```python
from build123d import *

# Parameters (mm, degrees)
SKETCH_1_R          = 48
SKETCH_1_R_2        = 40
EXTRUDE_1_DEPTH     = 8
SKETCH_2_R          = 45.05
SKETCH_2_R_2        = 42.95
CUT_EXTRUDE_1_DEPTH = 0.5
CUT_EXTRUDE_START   = -7.5
SKETCH_2_2_R        = 45.05
SKETCH_2_2_R_2      = 42.95
CUT_EXTRUDE_2_DEPTH = 0.5
CHAMFER_1_SIZE      = 0.8


with BuildPart() as part:
    # 草图1 → 凸台-拉伸1 (new body)
    with BuildSketch(Plane(origin=(0, 0, 0), x_dir=(1, 0, 0), z_dir=(0, 1, 0))):
        with Locations(Location((0, 0, 0), (0, 0, 270))):
            Circle(SKETCH_1_R)
        with Locations(Location((0, 0, 0), (0, 0, 270))):
            Circle(SKETCH_1_R_2, mode=Mode.SUBTRACT)
    extrude(amount=EXTRUDE_1_DEPTH)

    # 草图2 → 切除-拉伸1 (cut)
    with BuildSketch(Plane(origin=(0, 8, 0), x_dir=(1, 0, 0), z_dir=(0, 1, 0))):
        with Locations(Location((0, 0, 0), (0, 0, 270))):
            Circle(SKETCH_2_R)
        with Locations(Location((0, 0, 0), (0, 0, 270))):
            Circle(SKETCH_2_R_2, mode=Mode.SUBTRACT)
    extrude(amount=-CUT_EXTRUDE_1_DEPTH, mode=Mode.SUBTRACT)

    # 草图2<2> → 切除-拉伸2 (cut)
    with BuildSketch(Plane(origin=(0, 8, 0), x_dir=(1, 0, 0), z_dir=(0, 1, 0)).offset(CUT_EXTRUDE_START)):
        with Locations(Location((0, 0, 0), (0, 0, 270))):
            Circle(SKETCH_2_2_R)
        with Locations(Location((0, 0, 0), (0, 0, 270))):
            Circle(SKETCH_2_2_R_2, mode=Mode.SUBTRACT)
    extrude(amount=-CUT_EXTRUDE_2_DEPTH, mode=Mode.SUBTRACT)

    # 倒角1
    chamfer_1_edges = [part.edges().sort_by_distance(p)[0] for p in [
        (0, 0, -48),
        (0, 8, -48),
        (0, 0, -40),
        (0, 8, -40),
    ]]
    chamfer(chamfer_1_edges, length=CHAMFER_1_SIZE)


solid = part.part
```
Input: part model. Units: mm. Frame: model coordinates. A direction names the side the tool comes from. Round coordinates to 2 decimals unless told otherwise and drop trailing zeros. Order: outer loops, then holes, each group sorted by start corner. A loop starts at its lowest first (then second) coordinate and runs counter-clockwise, first axis right, second up. Notation, with made-up numbers: (58.5, -24) - (116.5, -24) arc R12 ccw to (116.5, -7) - close; hole circle Ø9 at (-17.75, -19.5). An arc over 180 degrees is marked (long way). One line per question, with ' | ' between items. Start each with the question number.
1) Ray query, probe 1 along X at (y, z) = (5, 0); probe 2 along X at (y, z) = (7.8, 0); probe 3 along X at (y, z) = (0.1, 0). Return the intervals inside material, ascending.
2) Contact query for flat-ended pins moving along their axis: P1, Ø4, axis at y = 5, z = 3, coming from the -X side; P2, Ø4, axis at y = 4.5, z = -34.5, coming from the +X side; P3, Ø1, axis at y = 4.5, z = 25, coming from the -X side. Output: stop coordinate, or through.
3) Pull-direction query (Z, two-part tool) for faces 4 (the cylindrical face through (14.418, 3.955, 45.783)), 5 (the flat face through (-17, 0, 42)), 6 (the cylindrical face through (13.53, 0.25, 42.97)); classes: +Z half, -Z half, draft (parallel to the pull), parting line (faces both ways), or undercut.
4) Set-up query: faces 1 (the flat face through (-16.47, 7.5, 39.83)), 2 (the cylindrical face through (-41.93, 0.25, -9.31)), 3 (the flat face through (-16, 8, 38)). Return all of +Z, -Z, +X, -X, +Y, -Y with unobstructed straight access to the full face (end or side cutting, diameter ignored); none if empty.
5) Cut plane C-C, the plane y = 5.5. Return the cut outline in (x, z), then the cut area to 3 significant figures.
Worked out:
1) probe 1: x = -48 to -40, 40 to 48 | probe 2: x = -47.4 to -45.05, -42.95 to -40.6, 40.6 to 42.95, 45.05 to 47.4 | probe 3: x = -47.3 to -45.05, -42.95 to -40.7, 40.7 to 42.95, 45.05 to 47.3
2) P1: stops at x = -47.99 | P2: stops at x = 35.32 | P3: stops at x = -41.28
3) face 4: parting line | face 5: draft | face 6: undercut
4) face 1: +Y | face 2: -Y | face 3: +Z, -Z, +X, -X, +Y
5) outline: circle Ø96 at (0, 0); hole circle Ø80 at (0, 0) | area: 2,210 mm^2
